```python
from build123d import *

# Parameters (mm, degrees)
SKETCH_1_W      = 39.5
SKETCH_1_H      = 20
EXTRUDE_1_DEPTH = 37
SKETCH_2_R      = 1.5
EXTRUDE_2_DEPTH = 9
SKETCH_14_W     = 15
SKETCH_14_H     = 1
EXTRUDE_5_DEPTH = 5
SKETCH_15_W     = 15
SKETCH_15_H     = 1
EXTRUDE_6_DEPTH = 5
M3X0_5_1_D      = 2.5
M3X0_5_1_DEPTH  = 8.5
M3X0_5_1_TIP    = 0.751075774
SKETCH_3_R      = 0.5
EXTRUDE_7_DEPTH = 2


with BuildPart() as part:
    # ｽｹｯﾁ1 → ﾎﾞｽ - 押し出し1 (new body)
    with BuildSketch(Plane(origin=(0, 0, 0), x_dir=(1, 0, 0), z_dir=(0, 1, 0))):
        with Locations((19.75, 10)):
            Rectangle(SKETCH_1_W, SKETCH_1_H)
    extrude(amount=EXTRUDE_1_DEPTH)

    # ｽｹｯﾁ2 → ﾎﾞｽ - 押し出し2 (add)
    with BuildSketch(Plane(origin=(0, 37, 0), x_dir=(1, 0, 0), z_dir=(0, 1, 0))):
        with Locations(Location((31, 10, 0), (0, 0, 90))):
            Circle(SKETCH_2_R)
    extrude(amount=EXTRUDE_2_DEPTH)

    # ｽｹｯﾁ14 → ﾎﾞｽ - 押し出し5 (add)
    with BuildSketch(Plane(origin=(39.5, 0, 0), x_dir=(0, 0, -1), z_dir=(1, 0, 0))):
        with Locations((10, 35.5)):
            Rectangle(SKETCH_14_W, SKETCH_14_H)
    extrude(amount=EXTRUDE_5_DEPTH)

    # ｽｹｯﾁ15 → ﾎﾞｽ - 押し出し6 (add)
    with BuildSketch(Plane.ZY):
        with Locations((-10, 35.5)):
            Rectangle(SKETCH_15_W, SKETCH_15_H)
    extrude(amount=EXTRUDE_6_DEPTH)

    # M3x0.5 ねじ穴1
    with Locations(Plane(origin=(0, 36, 0), x_dir=(1, 0, 0), z_dir=(0, 1, 0))):
        with Locations((-2.5, 13.5), (-2.5, 6.5), (42, 6.5), (42, 13.5)):
            Hole(M3X0_5_1_D / 2, depth=M3X0_5_1_DEPTH)
            with Locations((0, 0, -(M3X0_5_1_DEPTH + M3X0_5_1_TIP / 2))):  # 118° drill point
                Cone(0, M3X0_5_1_D / 2, M3X0_5_1_TIP, mode=Mode.SUBTRACT)

    # ｽｹｯﾁ3 → ﾎﾞｽ - 押し出し7 (add)
    with BuildSketch(Plane(origin=(0, 46, 0), x_dir=(1, 0, 0), z_dir=(0, 1, 0))):
        with Locations(Location((31, 10, 0), (0, 0, 270))):
            Circle(SKETCH_3_R)
    extrude(amount=EXTRUDE_7_DEPTH)


solid = part.part
```
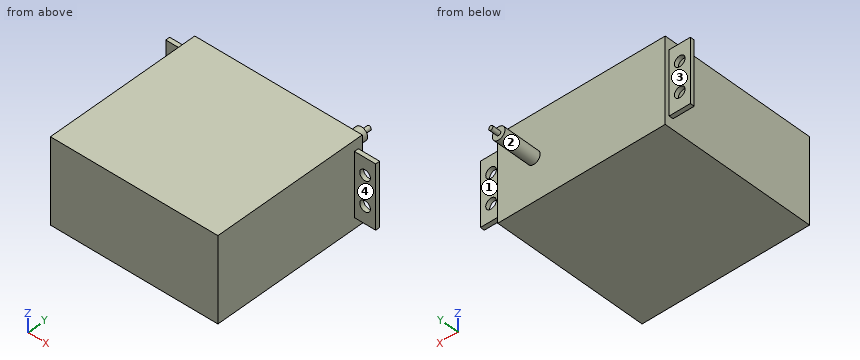
For this review, take the finished solid that the model builds, in its own axes (mm). Face numbers are marked on the shaded views. A direction names the side the tool comes from. Coordinates: 2 decimals unless noted, no trailing zeros. Order: outer loops, then holes, each group sorted by start corner. A loop starts at its lowest first (then second) coordinate and runs counter-clockwise, first axis right, second up. Notation, with made-up numbers: (5.5, -19) -> (31.5, -19) arc R19 cw to (31.5, -15) -> close; hole circle Ø6 at (64, -6.75). An arc over 180 degrees is marked (long way). Answer as CSV lines item,"result".
Q1. For the marked faces 1, 2, 3 and 4, list the 3-axis set-ups (+Z, -Z, +X, -X, +Y, -Y) from which the entire face can be reached by the end or side of a thin tool; tool diameter is ignored.
Model answer:
face 1,"+Z, -Z, +X, +Y"
face 2,"+Y"
face 3,"+Z, -Z, -X, +Y"
face 4,"+Z, -Z, +X, -Y"
Q2. Clearance check with flat-ended pins moving along their axes: pin 1 Ø12 at (x, z) = (33, -8) entering from +Y; pin 2 Ø10 at (x, z) = (24, -12) entering from +Y; pin 3 Ø0.5 at (x, y) = (42, 35.5) entering from +Z; pin 4 Ø2.5 at (x, z) = (-2.5, -10) entering from +Y. State where each tip first meets the part, or that it passes through.
Model answer:
pin 1,"stops at y = 48"
pin 2,"stops at y = 37"
pin 3,"stops at z = -2.5"
pin 4,"stops at y = 36"
Q3. We need section C-C (z = -16). State the section outline as (x, y) points, plus the area to 3 significant figures.
Model answer:
outline,"(-5, 35) -> (0, 35) -> (0, 0) -> (39.5, 0) -> (39.5, 35) -> (44.5, 35) -> (44.5, 36) -> (39.5, 36) -> (39.5, 37) -> (0, 37) -> (0, 36) -> (-5, 36) -> close"
area,"1,470 mm2"
Q4. Wall thickness on line 1 along X through (y, z) = (35.65, -6.5); line 2 along Z through (x, y) = (-2.5, 35.3); line 3 along X through (y, z) = (14, -10): over which ranges is each line inside the solid? List them lowest first. Write a range as [from, to].
Model answer:
line 1,"x = [-5, -3.75], [-1.25, 40.75], [43.25, 44.5]"
line 2,"z = [-17.5, -14.75], [-12.25, -7.75], [-5.25, -2.5]"
line 3,"x = [0, 39.5]"
Q5. We need section A-A (z = -6.5). State the section outline as (x, y) points, plus the area to 3 significant figures.
Model answer:
outline,"(-5, 35) -> (-3.75, 35) -> (-3.75, 36) -> (-5, 36) -> close; (-1.25, 35) -> (0, 35) -> (0, 0) -> (39.5, 0) -> (39.5, 35) -> (40.75, 35) -> (40.75, 36) -> (39.5, 36) -> (39.5, 37) -> (0, 37) -> (0, 36) -> (-1.25, 36) -> close; (43.25, 35) -> (44.5, 35) -> (44.5, 36) -> (43.25, 36) -> close"
area,"1,470 mm2"
Q6. We need section D-D (y = 17.5). State the section outline as (x, z) points.
Model answer:
outline,"(0, -20) -> (39.5, -20) -> (39.5, 0) -> (0, 0) -> close"
Q7. We need section B-B (x = 42). State the section outline as (y, z) points.
Model answer:
outline,"(35, -17.5) -> (36, -17.5) -> (36, -14.75) -> (35, -14.75) -> close; (35, -12.25) -> (36, -12.25) -> (36, -7.75) -> (35, -7.75) -> close; (35, -5.25) -> (36, -5.25) -> (36, -2.5) -> (35, -2.5) -> close"
